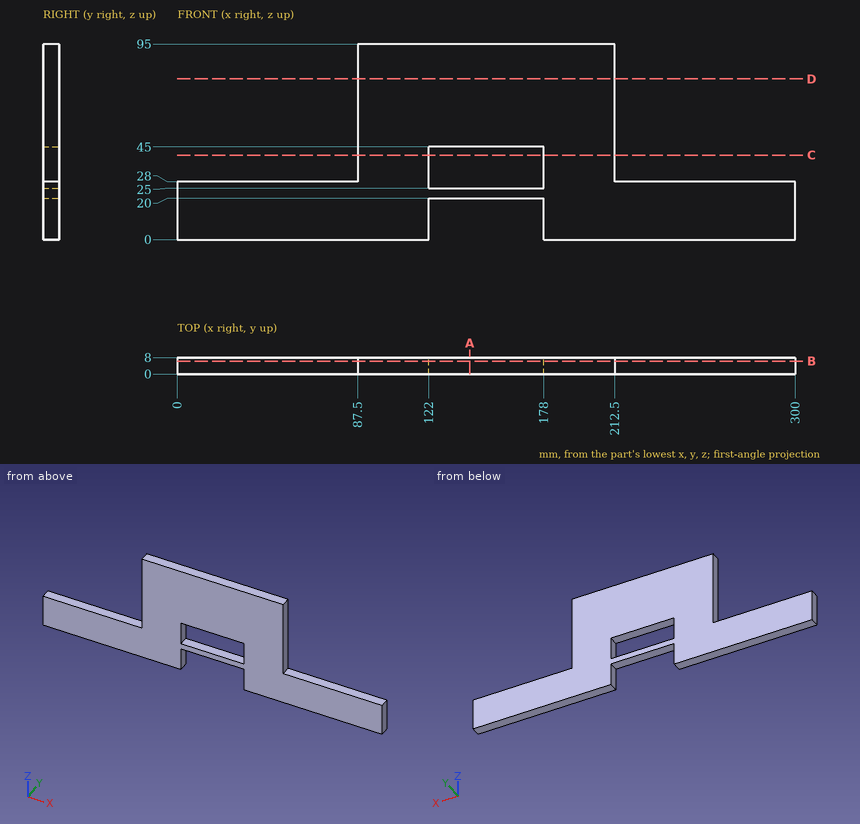
The figure shows three views and two pictorial views of one solid part (mm, origin at its lowest corner). Answer the questions. Give positions to 0.01 mm unless a question says otherwise; leave off trailing zeros. Write each loop counter-clockwise with the first axis right and the second up, starting at its lowest first coordinate (ties: lowest second). Pieces come first, ordered by that corner, then holes. Notation, with made-up numbers: (-29, 3.25) -> (30, 3.25) arc R11 cw to (30, 12.25) -> close; hole circle Ø6 at (-7, 38). An arc over 180 degrees is marked (long way). Answer as a JSON object with one key per item and string values.
1) Section B-B on y = 6.25 is taken. Write down the section's boundary in (x, z).
Findings below:
{"outline": "(0, 0) -> (122, 0) -> (122, 20) -> (178, 20) -> (178, 0) -> (300, 0) -> (300, 28) -> (212.5, 28) -> (212.5, 95) -> (87.5, 95) -> (87.5, 28) -> (0, 28) -> close; hole (122, 25) -> (178, 25) -> (178, 45) -> (122, 45) -> close"}
2) Flat-ended cylindrical pins translate along their axes: pin 1 Ø4 at (x, y) = (37, 3.5) entering from +Z; pin 2 Ø2.5 at (y, z) = (2, 56) entering from +X; pin 3 Ø4 at (y, z) = (5.5, 69) entering from -X. Find the tip coordinate at first contact, or state that the pin passes through.
Findings below:
{"pin 1": "stops at z = 28", "pin 2": "stops at x = 212.5", "pin 3": "stops at x = 87.5"}
3) Section D-D on z = 78 is taken. Write down the section's boundary in (x, y), then the cut area to 3 significant figures.
Findings below:
{"outline": "(87.5, 0) -> (212.5, 0) -> (212.5, 8) -> (87.5, 8) -> close", "area": "1,000 mm^2"}
4) Section C-C on z = 41 is taken. Write down the section's boundary in (x, y).
Findings below:
{"outline": "(87.5, 0) -> (122, 0) -> (122, 8) -> (87.5, 8) -> close; (178, 0) -> (212.5, 0) -> (212.5, 8) -> (178, 8) -> close"}
5) Section A-A on x = 142 is taken. Write down the section's boundary in (y, z).
Findings below:
{"outline": "(0, 20) -> (8, 20) -> (8, 25) -> (0, 25) -> close; (0, 45) -> (8, 45) -> (8, 95) -> (0, 95) -> close"}
6) Straight lines are drawn through the part: probe 1 along X at (y, z) = (7.5, 31.5); probe 2 along X at (y, z) = (4.75, 5.5); probe 3 along Z at (x, y) = (159, 1). For each, find the intervals that lie inside material, in ascending order. Write a range as from..to.
Findings below:
{"probe 1": "x = 87.5..122, 178..212.5", "probe 2": "x = 0..122, 178..300", "probe 3": "z = 20..25, 45..95"}
